The drawing under review shows one solid part. Ordinate dimensions are in mm from its lowest x, y, z. Give positions to 0.01 mm unless a question says otherwise; leave off trailing zeros. Order: outer loops, then holes, each group sorted by start corner. A loop starts at its lowest first (then second) coordinate and runs counter-clockwise, first axis right, second up. Notation, with made-up numbers: (5, 40) - (34, 40) arc R29 ccw to (34, 73) - close; hole circle Ø7 at (11, -33.75). An arc over 180 degrees is marked (long way). Use CSV: the item, a comma, the result in double quotes.
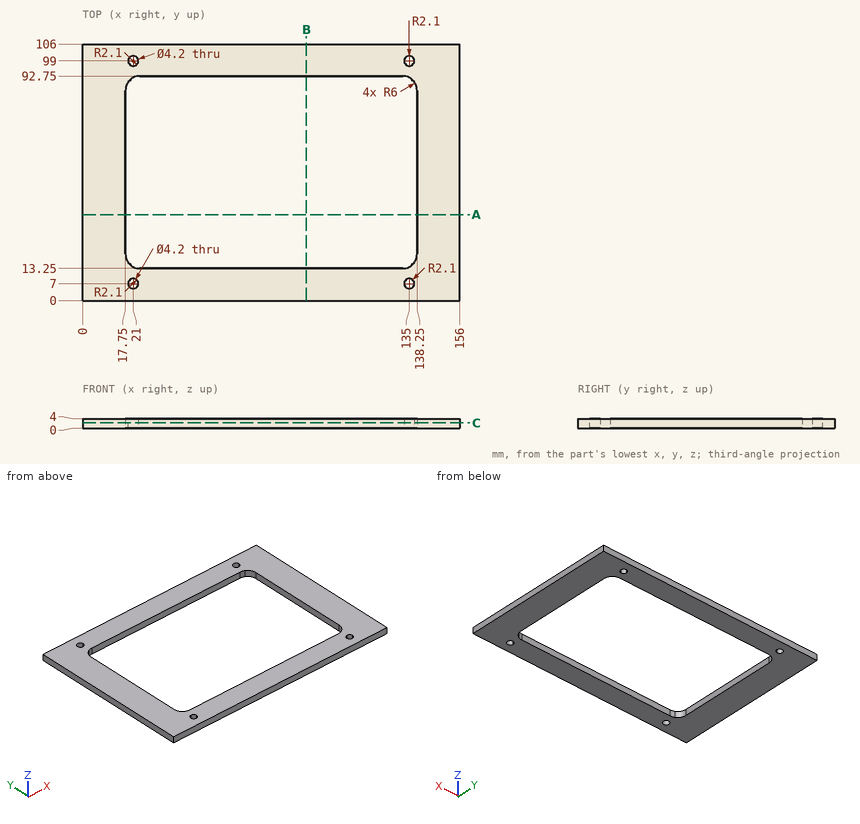
Item 1: Take a section at B-B, the plane x = 92.5. Give the boundary of the cut face in (y, z).
Results list:
outline,"(0, 0) - (13.25, 0) - (13.25, 4) - (0, 4) - close; (92.75, 0) - (106, 0) - (106, 4) - (92.75, 4) - close"
Item 2: Take a section at A-A, the plane y = 35.5. Give the boundary of the cut face in (x, z).
Results list:
outline,"(0, 0) - (17.75, 0) - (17.75, 4) - (0, 4) - close; (138.25, 0) - (156, 0) - (156, 4) - (138.25, 4) - close"
Item 3: Take a section at C-C, the plane z = 2.2. Give the boundary of the cut face in (x, y).
Results list:
outline,"(0, 0) - (156, 0) - (156, 106) - (0, 106) - close; hole (17.75, 19.25) arc R6 ccw to (23.75, 13.25) - (132.25, 13.25) arc R6 ccw to (138.25, 19.25) - (138.25, 86.75) arc R6 ccw to (132.25, 92.75) - (23.75, 92.75) arc R6 ccw to (17.75, 86.75) - close; hole circle Ø4.2 at (21, 7); hole circle Ø4.2 at (21, 99); hole circle Ø4.2 at (135, 7); hole circle Ø4.2 at (135, 99)"
Item 4: Wall thickness on L1, parallel to X at y = 7, z = 2.45; L2, parallel to Y at x = 21, z = 3.15; L3, parallel to Y at x = 51, z = 2.65: over which ranges is each line inside the solid? List them lowest first.
Results list:
L1,"x = 0 to 18.9, 23.1 to 132.9, 137.1 to 156"
L2,"y = 0 to 4.9, 9.1 to 13.92, 92.08 to 96.9, 101.1 to 106"
L3,"y = 0 to 13.25, 92.75 to 106"
